Source: CAD feature listing. Evaluate the final solid. Frame: model axes, mm. A direction names the side the tool comes from. Give positions to 0.01 mm unless a question says otherwise; leave off trailing zeros. Write each loop counter-clockwise with the first axis right and the second up, starting at its lowest first coordinate (ties: lowest second). Pieces come first, ordered by that corner, then holes. Notation, with made-up numbers: M -8.75,62 L 42.25,62 A28 ccw 42.25,83 Z; hole C -33.75,59.25 d8. An arc over 180 degrees is marked long. Use CSV: the item, a comma, the result in double quotes. Start each with the question number.
from build123d import *

# Parameters (mm, degrees)
F0_W     = 59.69
F0_H     = 117.856
F1_DEPTH = 4.572
F2_D     = 10.16
F3_D     = 5.08


with BuildPart() as f1:
    # F0 (on Front) → F1 (new body)
    with BuildSketch(Plane.XZ):
        Rectangle(F0_W, F0_H)
        with BuildLine():
            ThreePointArc((-1.7145, 45.72), (0, 47.4345), (1.7145, 45.72))
            Line((1.7145, 45.72), (1.7145, -25.908))
            ThreePointArc((1.7145, -25.908), (0, -27.6225), (-1.7145, -25.908))
            Line((-1.7145, -25.908), (-1.7145, 45.72))
        make_face(mode=Mode.SUBTRACT)
    extrude(amount=F1_DEPTH)

    # F2 (through all)
    with Locations(Plane(origin=(0, 0, 0), x_dir=(1, 0, 0), z_dir=(0, 1, 0))):
        with Locations((-19.431, -48.3362), (19.431, -48.3362), (23.3426, -25.527)):
            Hole(F2_D / 2)

    # F3 (through all)
    with Locations(Plane(origin=(0, 0, 0), x_dir=(1, 0, 0), z_dir=(0, 1, 0))):
        with Locations((-22.225, 0.762), (22.225, 0.762), (-15.875, 55.372), (15.875, 55.372)):
            Hole(F3_D / 2)


solid = f1.part
Item 1: Section C-C (y = -3.05). State how many separate pieces and enclosed holes the cut face has, plus the area to 3 significant figures.
Item 2: Pull-direction query (X, two-part tool) for faces 1 (the flat face through (-29.845, -2, -1)), 2 (the flat face through (1.714, -2, 10)), 3 (the flat face through (0, -2, 58.928)); classes: released by +X, released by -X, zero draft, split by the parting line, or undercut.
Item 3: Section B-B (x = 0). Return the cut outline in (y, z).
Item 4: Set-up query: faces 4 (the flat face through (-7, -4.572, 1)), 5 (the cylindrical face through (-0.038, -2.254, 47.434)). Return all of +Z, -Z, +X, -X, +Y, -Y with unobstructed straight access to the full face (end or side cutting, diameter ignored); none if empty.
Item 5: Section D-D (x = 21.5). Return the cut outline in (y, z).
Item 6: Section A-A (z = 34). Return the cut outline in (x, y) (1 decimal), plus the area to 3 significant figures.
Item 7: Material intervals for probe 1 along X at (y, z) = (-3.6, 18) (1 decimal); probe 2 along Z at (x, y) = (16.5, -2.8); probe 3 along Z at (x, y) = (-16, -0.7), sorted ascending.
Output values:
1,separate pieces,"1"
1,enclosed holes,"8"
1,area,"6,460 mm2"
2,face 1,"released by -X"
2,face 2,"undercut"
2,face 3,"zero draft"
3,outline,"M -4.57,-58.93 L 0,-58.93 L 0,-27.62 L -4.57,-27.62 Z; M -4.57,47.43 L 0,47.43 L 0,58.93 L -4.57,58.93 Z"
4,face 4,"+Z, -Z, +X, -X, -Y"
4,face 5,"+Y, -Y"
5,outline,"M -4.57,-58.93 L 0,-58.93 L 0,-3.2 L -4.57,-3.2 Z; M -4.57,1.67 L 0,1.67 L 0,20.79 L -4.57,20.79 Z; M -4.57,30.26 L 0,30.26 L 0,43.7 L -4.57,43.7 Z; M -4.57,52.98 L 0,52.98 L 0,58.93 L -4.57,58.93 Z"
6,outline,"M -29.8,-4.6 L -1.7,-4.6 L -1.7,0 L -29.8,0 Z; M 1.7,-4.6 L 29.8,-4.6 L 29.8,0 L 1.7,0 Z"
6,area,"257 mm2"
7,probe 1,"x = -29.8 to -1.7, 1.7 to 29.8"
7,probe 2,"z = -58.93 to -57.83, -52.91 to 44.19, 52.49 to 58.93"
7,probe 3,"z = -58.93 to -57.91, -52.84 to 44.59, 52.08 to 58.93"
